The listing builds one solid part. Answer for the finished solid, in the listing's coordinates (mm). A direction names the side the tool comes from. Give positions to 0.01 mm unless a question says otherwise; leave off trailing zeros. Write each loop counter-clockwise with the first axis right and the second up, starting at its lowest first coordinate (ties: lowest second). Pieces come first, ordered by that corner, then holes. Notation, with made-up numbers: (-30, -30) - (19, -30) arc R27 ccw to (19, -10) - close; hole circle Ø11 at (9, 87). An arc over 180 degrees is marked (long way). One line per question, with ' | ' between items. Start each with the question number.
1. For faces 1 (the face through (6, -48.5, 1)), 2 (the face through (0.43, -49.55, 0.99)), determine the directions among +Z, -Z, +X, -X, +Y, -Y from which every point of the face is accessible in a straight line to the end or side of a thin tool.
2. The mould has two halves that part along Z. Classify faces 3 (the face through (0.7, -24.9, 2)), 4 (the face through (0.7, -24.9, 0)), 5 (the face through (6, -50, 1)): +Z half, -Z half, draft (parallel to the pull), parting line (faces both ways), or undercut.
3. Find the intervals of material crossed by L1, parallel to X at y = -12.5, z = 0.8; L2, parallel to Y at x = 6.25, z = 1.6; L3, parallel to X at y = -21, z = 1.8, in increasing order. Write a range as from..to.
4. A cutting plane is placed at A-A (x = 8.25). Determine the outline of the cut face in (y, z).
5. Given P1, Ø0.5, axis at x = 4.5, z = 1, coming from the +Y side; P2, Ø0.8, axis at y = -18.5, z = 1, coming from the +X side; P3, Ø2, axis at x = 3.5, y = -5.5, coming from the +Z side, each flat-ended and moving along its own axis, determine where each tip first touches the part or whether it passes through.
6. A cutting plane is placed at C-C (y = -26). Determine the outline of the cut face in (x, z).
7. A cutting plane is placed at B-B (z = 1). Determine the outline of the cut face in (x, y), then the cut area to 3 significant figures.
```python
from build123d import *

# Parameters (mm, degrees)
F1_DEPTH    = 2
F2_T1_DEPTH = 9.5
F3_R        = 0.5


# Not quite as in the source:
# - a fillet or chamfer that OpenCascade refuses, or shapes differently, is made with other operations: its cross-section is extruded or revolved along the edge and cut away or added


with BuildPart() as f1:
    # F0 (on Top) → F1 (new body)
    with BuildSketch(Plane.XY):
        Polygon((1.5, 0), (0, 0), (0, -50), (11.5, -50), (11.5, -48.5), (1.5, -48.5), align=None)
    extrude(amount=F1_DEPTH)

    # F2: fillet of radius 1.5 on 3 edges, made by hand

    # F2_s2 → F2_t1 (cut)
    with BuildSketch(Plane.XY.offset(-3.75)):
        with BuildLine():
            ThreePointArc((10, -50), (11.0606601718, -49.5606601718), (11.5, -48.5))
            Line((11.5, -48.5), (11.5, -50))
            Line((11.5, -50), (10, -50))
        make_face()
        with BuildLine():
            ThreePointArc((0, -48.5), (0.4393398282, -49.5606601718), (1.5, -50))
            Line((1.5, -50), (0, -50))
            Line((0, -50), (0, -48.5))
        make_face()
        with BuildLine():
            ThreePointArc((11.5, -50), (11.0606601718, -48.9393398282), (10, -48.5))
            Line((10, -48.5), (11.5, -48.5))
            Line((11.5, -48.5), (11.5, -50))
        make_face()
    extrude(amount=F2_T1_DEPTH, mode=Mode.SUBTRACT)

    # F3
    f3_edges = [f1.edges().sort_by_distance(p)[0] for p in [
        (0, -24.25, 2),
        (0, -24.25, 0),
        (1.5, -24.25, 0),
        (1.5, -24.25, 2),
        (1.5, 0, 1),
        (0, 0, 1),
        (0.75, 0, 0),
        (0.75, 0, 2),
        (5.75, -48.5, 0),
        (10.75, -48.700962, 0),
        (10.75, -49.799038, 0),
        (5.75, -50, 0),
        (0.43934, -49.56066, 0),
        (5.75, -48.5, 2),
        (10.75, -48.700962, 2),
        (10.75, -49.799038, 2),
        (5.75, -50, 2),
        (0.43934, -49.56066, 2),
    ]]
    fillet(f3_edges, radius=F3_R)


solid = f1.part
```
Determined:
1) face 1: +Z, -Z, +X, +Y | face 2: +Z, -Z, -X, -Y
2) face 3: +Z half | face 4: -Z half | face 5: draft
3) L1: 0..1.5 | L2: -49.99..-48.51 | L3: 0.1..1.4
4) outline: (-50, 0.5) arc R0.5 ccw to (-49.5, 0) - (-49, 0) arc R0.5 ccw to (-48.5, 0.5) - (-48.5, 1.5) arc R0.5 ccw to (-49, 2) - (-49.5, 2) arc R0.5 ccw to (-50, 1.5) - close
5) P1: y = -48.5 | P2: x = 1.5 | P3: through
6) outline: (0, 0.5) arc R0.5 ccw to (0.5, 0) - (1, 0) arc R0.5 ccw to (1.5, 0.5) - (1.5, 1.5) arc R0.5 ccw to (1, 2) - (0.5, 2) arc R0.5 ccw to (0, 1.5) - close
7) outline: (0, -48.5) arc R1.5 ccw to (1.5, -50) - (10, -50) arc R1.5 ccw to (11.3, -49.25) arc R1.5 ccw to (10, -48.5) - (1.5, -48.5) - (1.5, -0.5) arc R0.5 ccw to (1, 0) - (0.5, 0) arc R0.5 ccw to (0, -0.5) - close | area: 88.5 mm2
